from build123d import *

# Parameters (mm, degrees)
SKETCH1_R           = 1
BOSS_EXTRUDE3_DEPTH = 1
SKETCH3_R           = 1
BOSS_EXTRUDE4_DEPTH = 1


with BuildPart() as part:
    # Sketch1 → Boss-Extrude3 (new body)
    with BuildSketch(Plane(origin=(0, 0, 0), x_dir=(1, 0, 0), z_dir=(0, 1, 0))):
        with BuildLine():
            Line((0.435948957, 3.056735566), (25.006928102, 2.999992))
            ThreePointArc((25.006928102, 2.999992), (27.999992, -0.006928102), (24.993071898, -2.999992))
            Line((24.993071898, -2.999992), (0.495326263, -2.943417558))
            ThreePointArc((0.495326263, -2.943417558), (0.15316776, -3.002934926), (-0.147999921, -3.175888058))
            Line((-0.147999921, -3.175888058), (-13.578162843, -14.392382292))
            ThreePointArc((-13.578162843, -14.392382292), (-14.642844141, -14.530674651), (-15.219179661, -13.624855459))
            ThreePointArc((-15.219179661, -13.624855459), (-16.155963413, 0.086416086), (-15.219179661, 13.797687632))
            ThreePointArc((-15.219179661, 13.797687632), (-14.640751142, 14.704482805), (-13.574624688, 14.562245599))
            Line((-13.574624688, 14.562245599), (-0.206296649, 3.292174932))
            ThreePointArc((-0.206296649, 3.292174932), (0.094068998, 3.117832635), (0.435948957, 3.056735566))
        make_face()
        with Locations((25, 0)):
            Circle(SKETCH1_R, mode=Mode.SUBTRACT)
    extrude(amount=BOSS_EXTRUDE3_DEPTH)

    # Sketch3 → Boss-Extrude4 (add)
    with BuildSketch(Plane.XZ):
        Circle(SKETCH3_R)
    extrude(amount=BOSS_EXTRUDE4_DEPTH)


solid = part.part
Verification items for the finished model (mm, model axes). A direction names the side the tool comes from. Round coordinates to 2 decimals unless told otherwise and drop trailing zeros. Write each loop counter-clockwise with the first axis right and the second up, starting at its lowest first coordinate (ties: lowest second). Pieces come first, ordered by that corner, then holes.
(1) Section check C-C (x = 17.5). Enter the section's corners in (y, z).
Returned:
outline: (0, -3.02) - (1, -3.02) - (1, 2.98) - (0, 2.98) - close
(2) Depth check by flat-ended pin: pin 1 Ø10 at (x, z) = (-3.5, -4) entering from -Y. Enter the tip coordinate at first touch or a pass-through.
Returned:
pin 1: stops at y = -1
(3) Material ranges on line 1 (Z direction, x = 25, y = 0.3); line 2 (X direction, y = 0.7, z = 0); line 3 (Y direction, x = 9, z = 1.5), recorded low to high.
Returned:
line 1: z = -3 to -1, 1 to 3
line 2: x = -16.16 to 24, 26 to 28
line 3: y = 0 to 1
(4) Section check A-A (y = 0.55). Enter the section's corners in (x, z).
Returned:
outline: (-15.22, -13.8) arc R1 ccw to (-13.57, -14.56) - (-0.21, -3.29) arc R1 cw to (0.44, -3.06) - (25.01, -3) arc R3 ccw to (24.99, 3) - (0.5, 2.94) arc R1 cw to (-0.15, 3.18) - (-13.58, 14.39) arc R1 ccw to (-15.22, 13.62) arc R100.81 ccw to start; hole circle Ø2 at (25, 0)
(5) Section check D-D (z = 10.75). Enter the section's corners in (x, y), plus the area to 3 significant figures.
Returned:
outline: (-15.57, 0) - (-9.22, 0) - (-9.22, 1) - (-15.57, 1) - close
area: 6.35 mm2
(6) Access from +Z, -Z, +X, -X, +Y, -Y to the whole of each face (thin tool, end or side, straight path). Record for faces 1 (the cylindrical face through (-0.217, -0.493, -0.976)), 2 (the cylindrical face through (-14.655, 0.493, -14.698)).
Returned:
face 1: -Y
face 2: -Z, +Y, -Y
(7) Section check B-B (z = 0). Enter the section's corners in (x, y).
Returned:
outline: (-16.16, 0) - (-1, 0) - (-1, -1) - (1, -1) - (1, 0) - (24, 0) - (24, 1) - (-16.16, 1) - close; (26, 0) - (28, 0) - (28, 1) - (26, 1) - close
